```python
from build123d import *

# Parameters (mm, degrees)
SKETCH1_R               = 7.5
BOSS_EXTRUDE1_DEPTH     = 58
SKETCH2_W               = 38
SKETCH2_H               = 30
CUT_EXTRUDE1_DEPTH      = 84.865217872
CUT_EXTRUDE1_DEPTH_BACK = 84.865217872
SKETCH3_W               = 16
SKETCH3_H               = 6
CUT_EXTRUDE4_DEPTH      = 84.865217872
CUT_EXTRUDE4_DEPTH_BACK = 84.865217872
SKETCH4_R               = 7
CUT_EXTRUDE5_DEPTH      = 100.435906681
CUT_EXTRUDE5_DEPTH_BACK = 100.435906681
CUT_EXTRUDE6_DEPTH      = 84.865217872
CUT_EXTRUDE6_DEPTH_BACK = 84.865217872
SKETCH9_R               = 7.5
CUT_EXTRUDE10_DEPTH     = 12
CUT_EXTRUDE12_DEPTH     = 6
CUT_EXTRUDE13_DEPTH     = 12
CUT_EXTRUDE14_DEPTH     = 6


with BuildPart() as part:
    # Sketch1 → Boss-Extrude1 (new body)
    with BuildSketch(Plane.XY):
        with BuildLine():
            Line((32.5, -19), (-32.5, -19))
            Line((-32.5, -19), (-32.5, 5))
            ThreePointArc((-32.5, 5), (-15.83939444, 16.82575695), (4.16060556, 21))
            Line((4.16060556, 21), (32.5, 21))
            Line((32.5, 21), (45.490381057, 13.5))
            Line((45.490381057, 13.5), (45.490381057, -11.5))
            Line((45.490381057, -11.5), (32.5, -19))
        make_face()
        with Locations(Location((0, 0, 0), (0, 0, 180))):
            Circle(SKETCH1_R, mode=Mode.SUBTRACT)
    extrude(amount=BOSS_EXTRUDE1_DEPTH)

    # Sketch2 → Cut-Extrude1 (cut, two sides)
    with BuildSketch(Plane(origin=(0, 21, 0), x_dir=(1, 0, 0), z_dir=(0, 1, 0))) as cut_extrude1_sk:
        with Locations((2.5, -29)):
            Rectangle(SKETCH2_W, SKETCH2_H)
    extrude(amount=CUT_EXTRUDE1_DEPTH, mode=Mode.SUBTRACT)
    extrude(cut_extrude1_sk.sketch, amount=-CUT_EXTRUDE1_DEPTH_BACK, mode=Mode.SUBTRACT)

    # Sketch3 → Cut-Extrude4 (cut, two sides)
    with BuildSketch(Plane(origin=(0, 21, 0), x_dir=(1, 0, 0), z_dir=(0, 1, 0))) as cut_extrude4_sk:
        with Locations((-24.5, -47)):
            Rectangle(SKETCH3_W, SKETCH3_H)
        with Locations((-24.5, -11)):
            Rectangle(SKETCH3_W, SKETCH3_H)
    extrude(amount=CUT_EXTRUDE4_DEPTH, mode=Mode.SUBTRACT)
    extrude(cut_extrude4_sk.sketch, amount=-CUT_EXTRUDE4_DEPTH_BACK, mode=Mode.SUBTRACT)


with BuildPart() as body_2:
    # of the pieces the cut leaves, the one that is kept (cut_extrude4_keep)
    add(part.part.solids().sort_by_distance((4.16060556, 21, 0))[0])

    # Sketch4 → Cut-Extrude5 (cut, two sides)
    with BuildSketch(Plane(origin=(45.490381057, 0, 0), x_dir=(0, 0, -1), z_dir=(1, 0, 0))) as cut_extrude5_sk:
        with Locations(Location((-29, 0, 0), (0, 0, 90))):
            Circle(SKETCH4_R)
    extrude(amount=CUT_EXTRUDE5_DEPTH, mode=Mode.SUBTRACT)
    extrude(cut_extrude5_sk.sketch, amount=-CUT_EXTRUDE5_DEPTH_BACK, mode=Mode.SUBTRACT)

    # Sketch6 → Cut-Extrude6 (cut, two sides)
    with BuildSketch(Plane(origin=(0, 21, 0), x_dir=(1, 0, 0), z_dir=(0, 1, 0))) as cut_extrude6_sk:
        Polygon((32.5, 0), (45.490381057, -12.990381057), (45.490381057, 0), align=None)
        Polygon((45.490381057, -45.009618943), (45.490381057, -58), (32.5, -58), align=None)
    extrude(amount=CUT_EXTRUDE6_DEPTH, mode=Mode.SUBTRACT)
    extrude(cut_extrude6_sk.sketch, amount=-CUT_EXTRUDE6_DEPTH_BACK, mode=Mode.SUBTRACT)

    # Sketch9 → Cut-Extrude10 (cut)
    with BuildSketch(Plane.XY.offset(58)):
        with BuildLine():
            Line((30.5, 19), (4.16060556, 19))
            ThreePointArc((4.16060556, 19), (-5.358778616, 18.046586751), (-14.5, 15.224221872))
            Line((-14.5, 15.224221872), (-14.5, -17))
            Line((-14.5, -17), (30.5, -17))
            Line((30.5, -17), (30.5, 19))
        make_face()
        with Locations(Location((0, 0, 0), (0, 0, 180))):
            Circle(SKETCH9_R, mode=Mode.SUBTRACT)
    extrude(amount=-CUT_EXTRUDE10_DEPTH, mode=Mode.SUBTRACT)

    # Sketch10 → Cut-Extrude12 (cut)
    with BuildSketch(Plane.XY.offset(58)):
        with BuildLine():
            Line((-14.5, 15.224221872), (-14.5, -17))
            Line((-14.5, -17), (-32.5, -17))
            Line((-32.5, -17), (-32.5, 3))
            ThreePointArc((-32.5, 3), (-24.178137204, 10.110658721), (-14.5, 15.224221872))
        make_face()
    extrude(amount=-CUT_EXTRUDE12_DEPTH, mode=Mode.SUBTRACT)

    # Sketch14 → Cut-Extrude13 (cut)
    with BuildSketch(Plane(origin=(0, 0, 0), x_dir=(-1, 0, 0), z_dir=(0, 0, -1))):
        with BuildLine():
            Line((14.5, -17), (14.5, 15.224221872))
            ThreePointArc((14.5, 15.224221872), (5.358778616, 18.046586751), (-4.16060556, 19))
            Line((-4.16060556, 19), (-30.5, 19))
            Line((-30.5, 19), (-30.5, -17))
            Line((-30.5, -17), (14.5, -17))
        make_face()
    extrude(amount=-CUT_EXTRUDE13_DEPTH, mode=Mode.SUBTRACT)

    # Sketch15 → Cut-Extrude14 (cut)
    with BuildSketch(Plane(origin=(0, 0, 0), x_dir=(-1, 0, 0), z_dir=(0, 0, -1))):
        with BuildLine():
            Line((14.5, 15.224221872), (14.5, -17))
            Line((14.5, -17), (32.5, -17))
            Line((32.5, -17), (32.5, 1.972887098))
            ThreePointArc((32.5, 1.972887098), (24.250830172, 9.618447449), (14.5, 15.224221872))
        make_face()
    extrude(amount=-CUT_EXTRUDE14_DEPTH, mode=Mode.SUBTRACT)


solid = body_2.part
```
Source: CAD feature listing. Evaluate the final solid. Frame: model axes, mm. A direction names the side the tool comes from. Round coordinates to 2 decimals unless told otherwise and drop trailing zeros. Loops run counter-clockwise (first coordinate to the right, second up) from the corner with the lowest first, then second, coordinate; pieces in that order, holes last.
1. Mould query, pull axis Y, two halves, no side actions, for faces 1 (the flat face through (6, 6, 14)), 2 (the flat face through (-23, -4, 6)), 3 (the cylindrical face through (-4.032, -6.324, 12.986)), 4 (the cylindrical face through (-11.84, 18.37, 5.35)). Classes: released by +Y, released by -Y, zero draft, split by the parting line, or undercut.
2. Section query D-D on x = 0. Output: boundary loops of the cut face in (y, z), and give its area (3 significant figures).
3. Access query for faces 5 (the cylindrical face through (-11.84, 18.37, 52.46)), 6 (the cylindrical face through (-24.378, 9.525, 2.958)), 7 (the flat face through (8, 1, 46)), 8 (the flat face through (6, 6, 44)). Directions: +Z, -Z, +X, -X, +Y, -Y. A direction counts if a zero-diameter tool reaches every point of the face in a straight line with its end or side. Return the directions, or none.
4. Ray query, L1, parallel to Z at x = -9.5, y = -7; L2, parallel to Z at x = 37, y = 0; L3, parallel to X at y = -10, z = 16.5. Return the intervals inside material, ascending.
5. Section query B-B on y = 0. Give the number of separate pieces and of enclosed holes in the cut face, and give its area (3 significant figures).
6. Section query C-C on x = -20. Output: boundary loops of the cut face in (y, z), and give its area (3 significant figures).
7. Section query A-A on z = 29. Output: boundary loops of the cut face in (x, y).
8. Contact query for flat-ended pins moving along their axis: pin 1 (1.5 mm diameter, centred on y = 3, z = 9.5, fed in from +X); pin 2 (1 mm diameter, centred on x = 0.5, y = 14, fed in from -Z); pin 3 (12.5 mm diameter, centred on y = 0, z = 29, fed in from +X); pin 4 (18 mm diameter, centred on x = 5, y = 1.5, fed in from +Z). Output: stop coordinate, or through.
Answers below:
1. face 1: zero draft
1. face 2: undercut
1. face 3: undercut
1. face 4: released by +Y
2. outline: (-19, 0) - (-17, 0) - (-17, 12) - (-7.5, 12) - (-7.5, 14) - (-19, 14) - close; (-19, 44) - (-7.5, 44) - (-7.5, 46) - (-17, 46) - (-17, 58) - (-19, 58) - close; (7.5, 12) - (18.82, 12) - (18.82, 0) - (20.83, 0) - (20.83, 14) - (7.5, 14) - close; (7.5, 44) - (20.83, 44) - (20.83, 58) - (18.82, 58) - (18.82, 46) - (7.5, 46) - close
2. area: 195 mm2
3. face 5: +Z, -Z, -X, +Y
3. face 6: -Z
3. face 7: +Z
3. face 8: -X, +Y, -Y
4. L1: z = 12 to 14, 44 to 46
4. L2: z = 4.5 to 22, 36 to 53.5
4. L3: x = 21.5 to 45.49
5. separate pieces: 4
5. enclosed holes: 0
5. area: 851 mm2
6. outline: (-19, 0) - (-17, 0) - (-17, 6) - (12.43, 6) - (12.43, 0) - (14.78, 0) - (14.78, 8) - (-19, 8) - close; (-19, 50) - (14.78, 50) - (14.78, 58) - (12.66, 58) - (12.66, 52) - (-17, 52) - (-17, 58) - (-19, 58) - close
6. area: 186 mm2
7. outline: (21.5, -19) - (32.5, -19) - (45.49, -11.5) - (45.49, -7) - (21.5, -7) - close; (21.5, 7) - (45.49, 7) - (45.49, 13.5) - (32.5, 21) - (21.5, 21) - close
8. pin 1: stops at x = 42.75
8. pin 2: stops at z = 12
8. pin 3: passes through
8. pin 4: stops at z = 46
